Geometry: see drawing. Coordinates: mm, zero at the bounding-box minimum. Give positions to 0.01 mm unless a question says otherwise; leave off trailing zeros. Write each loop counter-clockwise with the first axis right and the second up, starting at its lowest first coordinate (ties: lowest second). Pieces come first, ordered by that corner, then holes.
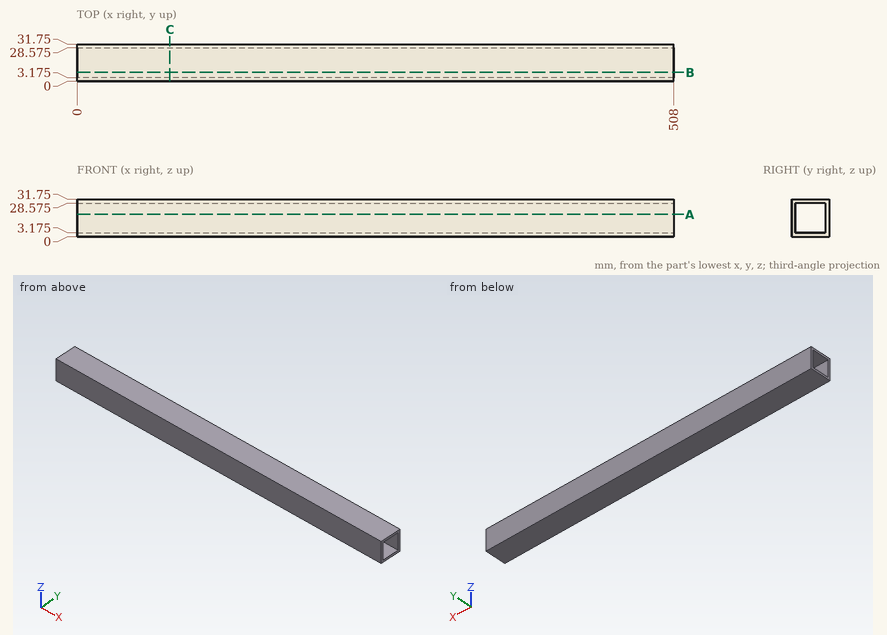
1. Section query C-C (x = 79). Return loops of the section in (y, z) (3 decimals).
2. Line query: probe 1 along Y at (x, z) = (408.5, 15) (3 decimals). Output: solid intervals per line, ascending.
3. Section query A-A (z = 19). Return loops of the section in (x, y) (3 decimals).
The answers:
1. outline: (0, 0) - (31.75, 0) - (31.75, 31.75) - (0, 31.75) - close; hole (3.175, 3.175) - (28.575, 3.175) - (28.575, 28.575) - (3.175, 28.575) - close
2. probe 1: y = 0 to 3.175, 28.575 to 31.75
3. outline: (0, 0) - (508, 0) - (508, 3.175) - (0, 3.175) - close; (0, 28.575) - (508, 28.575) - (508, 31.75) - (0, 31.75) - close
